For this review, take the finished solid that the model builds, in its own axes (mm). Give positions to 0.01 mm unless a question says otherwise; leave off trailing zeros. Write each loop counter-clockwise with the first axis right and the second up, starting at its lowest first coordinate (ties: lowest second). Pieces come first, ordered by that corner, then holes.
1) Wall thickness on line 1 along X through (y, z) = (-24.75, 1.95); line 2 along X through (y, z) = (-32.5, 0.7); line 3 along Y through (x, z) = (-16, 1.65): over which ranges is each line inside the solid? List them lowest first.
2) We need section C-C on z = 0.45. Give the boundary of the cut face in (x, y), and give its area (3 significant figures).
3) We need section D-D on y = -37.25. Give the boundary of the cut face in (x, z), and give its area (3 significant figures).
4) We need section A-A on y = -23.75. Give the boundary of the cut face in (x, z), and give its area (3 significant figures).
5) We need section B-B on x = -9. Give the boundary of the cut face in (y, z).
6) Draft analysis for pull direction Y (two halves, no side actions). For faces 1 (the face through (-5, -30, 2.5)), 2 (the face through (15.2, -27.9, 1.2)), 3 (the face through (-11, -39.141, 1)), state which applies: pulls with the +Y half, pulls with the -Y half, needs draft (parallel to the pull), parting line crosses it, or undercut.
7) For P1, Ø1.5, axis at y = -31, z = 1, coming from the -X side, flat-tipped, find the tip position at first contact; note if it passes through.
from build123d import *

# Parameters (mm, degrees)
F0_R     = 6.25
F1_DEPTH = 2.5


with BuildPart() as f1:
    # F0 (on Top) → F1 (new body)
    with BuildSketch(Plane.XY):
        with BuildLine():
            ThreePointArc((-28.549118, -16.640839), (-39.799118, -27.890839), (-28.549118, -39.140839))
            Line((-28.549118, -39.140839), (6.450882, -39.140839))
            ThreePointArc((6.450882, -39.140839), (13.472693, -36.680417), (17.423104, -30.375359))
            ThreePointArc((17.423104, -30.375359), (15.200882, -27.890839), (17.423104, -25.406319))
            ThreePointArc((17.423104, -25.406319), (13.472693, -19.101262), (6.450882, -16.640839))
            Line((6.450882, -16.640839), (-28.549118, -16.640839))
        make_face()
        with Locations((-11.049118, -27.890839)):
            Circle(F0_R, mode=Mode.SUBTRACT)
    extrude(amount=F1_DEPTH)


solid = f1.part
Results list:
1. line 1: x = -39.35 to -16.45, -5.65 to 17.25
1. line 2: x = -38.81 to -15.27, -6.83 to 16.71
1. line 3: y = -39.14 to -31.71, -24.08 to -16.64
2. outline: (-28.55, -39.14) - (6.45, -39.14) arc R11.25 ccw to (17.42, -30.38) arc R2.5 cw to (17.42, -25.41) arc R11.25 ccw to (6.45, -16.64) - (-28.55, -16.64) arc R11.25 ccw to start; hole circle Ø12.5 at (-11.05, -27.89)
2. area: 1,050 mm2
3. outline: (-34.79, 0) - (12.69, 0) - (12.69, 2.5) - (-34.79, 2.5) - close
3. area: 119 mm2
4. outline: (-39.01, 0) - (-15.73, 0) - (-15.73, 2.5) - (-39.01, 2.5) - close; (-6.37, 0) - (16.91, 0) - (16.91, 2.5) - (-6.37, 2.5) - close
4. area: 116 mm2
5. outline: (-39.14, 0) - (-33.8, 0) - (-33.8, 2.5) - (-39.14, 2.5) - close; (-21.99, 0) - (-16.64, 0) - (-16.64, 2.5) - (-21.99, 2.5) - close
6. face 1: needs draft
6. face 2: undercut
6. face 3: pulls with the -Y half
7. P1: stops at x = -39.55
